Model file for the job. Use its own axes, mm. Give positions to 0.01 mm unless a question says otherwise; leave off trailing zeros. Write each loop counter-clockwise with the first axis right and the second up, starting at its lowest first coordinate (ties: lowest second). Pieces come first, ordered by that corner, then holes. Notation, with made-up numbers: M 63.5,-8.5 L 113.5,-8.5 A18 ccw 113.5,3.5 Z; hole C 9,37 d11. An arc over 180 degrees is marked long. Answer as a JSON object with one key per item and string values. Group by question number.
Autodesk Inventor part; units mm, degrees
ref_plane "YZ Plane" through (0, 0, 0) normal (1, 0, 0) x (0, 1, 0)
ref_plane "XZ Plane" through (0, 0, 0) normal (0, 1, 0) x (-1, 0, 0)
ref_plane "XY Plane" through (0, 0, 0) normal (0, 0, 1) x (1, 0, 0)
sketch "Sketch1" plane through (0, 0, 0) normal (0, 0, 1) x (1, 0, 0)
  line L0 (29, 35) -> (-29, 35)
  line L1 (-29, 35) -> (-29, 20)
  line L2 (-29, 20) -> (-34, 20)
  line L3 (-34, 20) -> (-34, 0)
  line L4 (-34, 0) -> (-29, 0)
  line L5 (-29, 0) -> (-29, -35)
  line L6 (-29, -35) -> (29, -35)
  line L7 (31, -33) -> (31, 33)
  arc A0 (31, 33) -> (29, 35) centre (29, 33) ccw
  arc A1 (29, -35) -> (31, -33) centre (29, -33) ccw
  point P0 (0, 0)
  point P1 (31, 35)
  point P2 (31, -35)
  point P3 (31, 0)
  point P4 (0, 35)
  dimension "d0" = 70
  dimension "d1" = 5
  dimension "d2" = 20
  dimension "d3" = 15
  dimension "d4" = 60
  dimension "d7" = 2
extrude "Extrusion1" add sketch "Sketch1" along normal blind 5
sketch "Sketch2" plane through (0, 0, 5) normal (0, 0, 1) x (1, 0, 0)
  line L0 (-29, 35) -> (-29, 20)
  point P0 (0, 0)
  point P1 (-8, 5)
  dimension "d8" = 5
  dimension "d33" = 21
hole "Hole1" at (-8, 5, 5) direction (0, 0, -1) diameter 22 depth 8 tip angle 118
sketch "Sketch3" plane through (0, 0, 5) normal (0, 0, 1) x (1, 0, 0)
  circle A0 centre (-8, 5) radius 11
  line L0 (-23.5, -10.5) -> (7.5, -10.5) construction
  line L1 (7.5, -10.5) -> (7.5, 20.5) construction
  line L2 (7.5, 20.5) -> (-23.5, 20.5) construction
  line L3 (-23.5, 20.5) -> (-23.5, -10.5) construction
  line L4 (-23.5, -10.5) -> (7.5, 20.5) construction
  line L5 (7.5, -10.5) -> (-23.5, 20.5) construction
  point P0 (0, 0)
  dimension "d17" = 31
  dimension "d18" = 31
hole "Hole2" at (-23.5, 20.5, 5) at (7.5, 20.5, 5) at (7.5, -10.5, 5) at (-23.5, -10.5, 5) direction (0, 0, -1) diameter 3.4 depth 8 tip angle 118
sketch "Sketch4" plane through (0, 0, 5) normal (0, 0, 1) x (1, 0, 0)
  line L0 (-29, 20) -> (-29, 35)
  line L1 (-29, 30.25) -> (-24, 30.25)
  line L2 (-24, 30.25) -> (-24, 31.5)
  line L3 (-24, 31.5) -> (-20.8, 31.5)
  line L4 (-20.8, 31.5) -> (-20.8, 24.5)
  line L5 (-20.8, 24.5) -> (-24, 24.5)
  line L6 (-24, 24.5) -> (-24, 25.75)
  line L7 (-24, 25.75) -> (-29, 25.75)
  line L8 (-29, 25.75) -> (-29, 30.25)
  line L9 (-29, 20) -> (-34, 20)
  line L10 (-29, -6.4) -> (-24, -6.4)
  line L11 (-24, -6.4) -> (-24, -4.5)
  line L12 (-24, -4.5) -> (-20.8, -4.5)
  line L13 (-20.8, -4.5) -> (-20.8, -11.5)
  line L14 (-20.8, -11.5) -> (-24, -11.5)
  line L15 (-24, -11.5) -> (-24, -9.6)
  line L16 (-24, -9.6) -> (-29, -9.6)
  line L17 (-29, -9.6) -> (-29, -6.4)
  line L18 (-29, -35) -> (-29, 0)
  line L19 (-34, 0) -> (-29, 0)
  point P0 (0, 0)
  point P1 (-29, 28)
  point P2 (-20.8, 28)
  point P3 (-20.8, -8)
  point P4 (-29, -8)
  dimension "d37" = 7
  dimension "d38" = 3.2
  dimension "d39" = 5
  dimension "d42" = 4.5
  dimension "d43" = 8
  dimension "d44" = 7
  dimension "d45" = 3.2
  dimension "d46" = 5
  dimension "d47" = 3.2
  dimension "d48" = 8
extrude "Extrusion2" cut sketch "Sketch4" against normal blind 5
sketch "Sketch5" plane through (0, 0, 5) normal (0, 0, 1) x (1, 0, 0)
  line L0 (-5, -25) -> (5, -25)
  line L1 (5, -25) -> (5, -20)
  line L2 (5, -20) -> (-5, -20)
  line L3 (-5, -20) -> (-5, -25)
  line L4 (-5, -25) -> (5, -20) construction
  line L5 (5, -25) -> (-5, -20) construction
  line L6 (-29, -35) -> (29, -35)
  point P0 (0, 0)
  point P1 (0, -22.5)
  point P2 (0, -22.5)
  dimension "d28" = 10
  dimension "d29" = 5
  dimension "d34" = 10
extrude "Extrusion3" cut sketch "Sketch5" against normal blind 5
properties part number "Belt_Holder2" material "Polycarbonate, Clear"
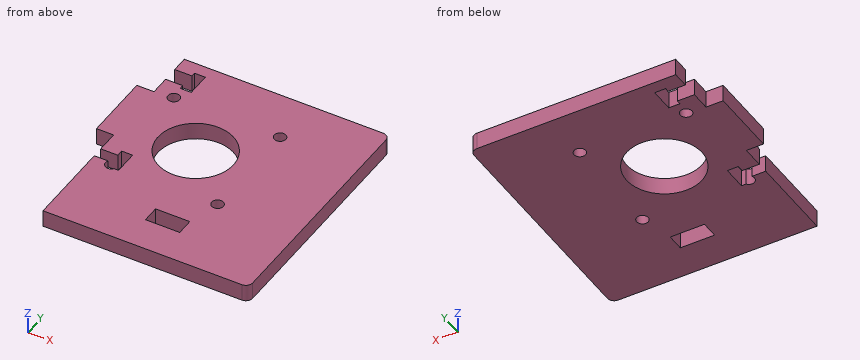
Q1. Wall check: L1, parallel to X at y = -10.5, z = 3.15; L2, parallel to X at y = 20.5, z = 2.8; L3, parallel to Y at x = 7.5, z = 2.75. Give the ranges that are in metal, low to high.
Q2. Slice it at A-A, the plane x = 7.5. Write the cut outline in (y, z).
Q3. Slice it at D-D, the plane x = -8. Write the cut outline in (y, z), then the cut area to 3 significant figures.
Q4. Drop flat-ended pins along their axis: P1, Ø2.5, axis at y = -9, z = 2.5, coming from the -X side; P2, Ø1.5, axis at y = -8.5, z = 0.5, coming from the -X side; P3, Ø2.5, axis at x = -31, z = 3.5, coming from the +Y side. Give the stop position or say it passes through.
Q5. Slice it at B-B, the plane z = 4. Count the separate pieces of the cut face and the enclosed holes in it, then the cut area to 3 significant figures.
Q6. Slice it at C-C, the plane y = -10.5. Write the cut outline in (x, z), then the cut area to 3 significant figures.
Solved:
{
 "1": {"L1": "x = -29 to -25.2, -20.8 to 5.8, 9.2 to 31", "L2": "x = -29 to -25.2, -21.8 to 5.8, 9.2 to 31", "L3": "y = -35 to -12.2, -8.8 to 18.8, 22.2 to 35"},
 "2": {"outline": "M -35,0 L -12.2,0 L -12.2,5 L -35,5 Z; M -8.8,0 L 18.8,0 L 18.8,5 L -8.8,5 Z; M 22.2,0 L 35,0 L 35,5 L 22.2,5 Z"},
 "3": {"outline": "M -35,0 L -6,0 L -6,5 L -35,5 Z; M 16,0 L 35,0 L 35,5 L 16,5 Z", "area": "240 mm²"},
 "4": {"P1": "stops at x = -29", "P2": "stops at x = -20.8", "P3": "stops at y = 20"},
 "5": {"separate pieces": "1", "enclosed holes": "5", "area": "3,750 mm²"},
 "6": {"outline": "M -29,0 L -25.2,0 L -25.2,5 L -29,5 Z; M -20.8,0 L 5.8,0 L 5.8,5 L -20.8,5 Z; M 9.2,0 L 31,0 L 31,5 L 9.2,5 Z", "area": "261 mm²"}
}
